from build123d import *

# Parameters (mm, degrees)
F0_W         = 150
F0_H         = 150
F1_DEPTH     = 50
F2_W         = 130.2189305425
F2_H         = 127.2944062948
F3_DEPTH     = 45
F4_T1_DEPTH  = 175.4
F4_T3_DEPTH  = 175.4
F4_T5_DEPTH  = 127.2944062948
F4_T7_DEPTH  = 130.2189305425
F4_T13_DEPTH = 142.9189305425
F4_T17_DEPTH = 139.9944062948
F4_T24_DEPTH = 139.9944062948
F4_T28_DEPTH = 142.9189305425
F4_T35_DEPTH = 139.9944062948
F4_T39_DEPTH = 142.9189305425
F4_T46_DEPTH = 139.9944062948
F4_T50_DEPTH = 142.9189305425


# Not quite as in the source:
# - a fillet or chamfer that OpenCascade refuses, or shapes differently, is made with other operations: its cross-section is extruded or revolved along the edge and cut away or added


with BuildPart() as f1:
    # F0 (on Top) → F1 (new body)
    with BuildSketch(Plane.XY):
        Rectangle(F0_W, F0_H)
    extrude(amount=F1_DEPTH)

    # F2 (on face) → F3 (cut)
    with BuildSketch(Plane.XY.offset(50)):
        with Locations((0.9621791542, 0.0429600477)):
            Rectangle(F2_W, F2_H)
    extrude(amount=-F3_DEPTH, mode=Mode.SUBTRACT)

    # F4: fillet of radius 5.08 on 8 edges, made by hand

    # F4_s2 → F4_t1 (cut)
    with BuildSketch(Plane.YZ.offset(-87.7)):
        with BuildLine():
            ThreePointArc((69.92, 50), (73.5121024484, 48.5121024484), (75, 44.92))
            Line((75, 44.92), (75, 50))
            Line((75, 50), (69.92, 50))
        make_face()
        with BuildLine():
            ThreePointArc((-75, 44.92), (-73.5121024484, 48.5121024484), (-69.92, 50))
            Line((-69.92, 50), (-75, 50))
            Line((-75, 50), (-75, 44.92))
        make_face()
    extrude(amount=F4_T1_DEPTH, mode=Mode.SUBTRACT)

    # F4_s4 → F4_t3 (cut)
    with BuildSketch(Plane.XZ.offset(-87.7)):
        with BuildLine():
            ThreePointArc((-75, 44.92), (-73.5121024484, 48.5121024484), (-69.92, 50))
            Line((-69.92, 50), (-75, 50))
            Line((-75, 50), (-75, 44.92))
        make_face()
        with BuildLine():
            ThreePointArc((75, 44.92), (73.5121024484, 48.5121024484), (69.92, 50))
            Line((69.92, 50), (75, 50))
            Line((75, 50), (75, 44.92))
        make_face()
    extrude(amount=F4_T3_DEPTH, mode=Mode.SUBTRACT)

    # F4_s6 → F4_t5 (cut)
    with BuildSketch(Plane.XZ.offset(-63.6901631951)):
        with BuildLine():
            ThreePointArc((71.1516444254, 50), (67.559541977, 48.5121024484), (66.0716444254, 44.92))
            Line((66.0716444254, 44.92), (66.0716444254, 50))
            Line((66.0716444254, 50), (71.1516444254, 50))
        make_face()
        with BuildLine():
            ThreePointArc((-69.2272861171, 50), (-65.6351836686, 48.5121024484), (-64.1472861171, 44.92))
            Line((-64.1472861171, 44.92), (-64.1472861171, 50))
            Line((-64.1472861171, 50), (-69.2272861171, 50))
        make_face()
    extrude(amount=F4_T5_DEPTH, mode=Mode.SUBTRACT)

    # F4_s8 → F4_t7 (cut)
    with BuildSketch(Plane.YZ.offset(-64.1472861171)):
        with BuildLine():
            ThreePointArc((-68.6842430997, 50), (-65.0921406513, 48.5121024484), (-63.6042430997, 44.92))
            Line((-63.6042430997, 44.92), (-63.6042430997, 50))
            Line((-63.6042430997, 50), (-68.6842430997, 50))
        make_face()
        with BuildLine():
            ThreePointArc((68.7701631951, 50), (65.1780607467, 48.5121024484), (63.6901631951, 44.92))
            Line((63.6901631951, 44.92), (63.6901631951, 50))
            Line((63.6901631951, 50), (68.7701631951, 50))
        make_face()
    extrude(amount=F4_T7_DEPTH, mode=Mode.SUBTRACT)


with BuildPart() as f4_tool11:
    # F4_s12 → F4_t13 (new body)
    with BuildSketch(Plane.YZ.offset(-64.1472861171)):
        with BuildLine():
            ThreePointArc((-68.6842430997, 50), (-65.0921406513, 48.5121024484), (-63.6042430997, 44.92))
            Line((-63.6042430997, 44.92), (-63.6042430997, 50))
            Line((-63.6042430997, 50), (-68.6842430997, 50))
        make_face()
    extrude(amount=F4_T13_DEPTH)

    split(bisect_by=Plane.YZ.offset(66.0716444254), keep=Keep.TOP)


with BuildPart() as f4_tool15:
    # F4_s16 → F4_t17 (new body)
    with BuildSketch(Plane.XZ.offset(76.3042430997)):
        with BuildLine():
            ThreePointArc((71.1516444254, 50), (67.559541977, 48.5121024484), (66.0716444254, 44.92))
            Line((66.0716444254, 44.92), (66.0716444254, 50))
            Line((66.0716444254, 50), (71.1516444254, 50))
        make_face()
    extrude(amount=-F4_T17_DEPTH)

    split(bisect_by=Plane.XZ.offset(63.6042430997), keep=Keep.TOP)


with BuildPart() as f4_tool11_1:
    add(f4_tool11.part)

    # F4_t19: intersect F4_tool15
    add(f4_tool15.part, mode=Mode.INTERSECT)


with BuildPart() as f1_1:
    add(f1.part)

    # F4_t9: cut F4_tool11
    add(f4_tool11_1.part, mode=Mode.SUBTRACT)


with BuildPart() as f4_tool22:
    # F4_s23 → F4_t24 (new body)
    with BuildSketch(Plane.XZ.offset(63.6042430997)):
        with BuildLine():
            ThreePointArc((71.1516444254, 50), (67.559541977, 48.5121024484), (66.0716444254, 44.92))
            Line((66.0716444254, 44.92), (66.0716444254, 50))
            Line((66.0716444254, 50), (71.1516444254, 50))
        make_face()
    extrude(amount=-F4_T24_DEPTH)

    split(bisect_by=Plane.XZ.offset(-63.6901631951), keep=Keep.BOTTOM)


with BuildPart() as f4_tool26:
    # F4_s27 → F4_t28 (new body)
    with BuildSketch(Plane.YZ.offset(78.7716444254)):
        with BuildLine():
            ThreePointArc((68.7701631951, 50), (65.1780607467, 48.5121024484), (63.6901631951, 44.92))
            Line((63.6901631951, 44.92), (63.6901631951, 50))
            Line((63.6901631951, 50), (68.7701631951, 50))
        make_face()
    extrude(amount=-F4_T28_DEPTH)

    split(bisect_by=Plane.YZ.offset(66.0716444254), keep=Keep.TOP)


with BuildPart() as f4_tool22_1:
    add(f4_tool22.part)

    # F4_t30: intersect F4_tool26
    add(f4_tool26.part, mode=Mode.INTERSECT)


with BuildPart() as f1_2:
    add(f1_1.part)

    # F4_t20: cut F4_tool22
    add(f4_tool22_1.part, mode=Mode.SUBTRACT)


with BuildPart() as f4_tool33:
    # F4_s34 → F4_t35 (new body)
    with BuildSketch(Plane.XZ.offset(-63.6901631951)):
        with BuildLine():
            ThreePointArc((-69.2272861171, 50), (-65.6351836686, 48.5121024484), (-64.1472861171, 44.92))
            Line((-64.1472861171, 44.92), (-64.1472861171, 50))
            Line((-64.1472861171, 50), (-69.2272861171, 50))
        make_face()
    extrude(amount=F4_T35_DEPTH)

    split(bisect_by=Plane.XZ.offset(63.6042430997), keep=Keep.TOP)


with BuildPart() as f4_tool37:
    # F4_s38 → F4_t39 (new body)
    with BuildSketch(Plane.YZ.offset(-76.8472861171)):
        with BuildLine():
            ThreePointArc((-68.6842430997, 50), (-65.0921406513, 48.5121024484), (-63.6042430997, 44.92))
            Line((-63.6042430997, 44.92), (-63.6042430997, 50))
            Line((-63.6042430997, 50), (-68.6842430997, 50))
        make_face()
    extrude(amount=F4_T39_DEPTH)

    split(bisect_by=Plane.YZ.offset(-64.1472861171), keep=Keep.BOTTOM)


with BuildPart() as f4_tool33_1:
    add(f4_tool33.part)

    # F4_t41: intersect F4_tool37
    add(f4_tool37.part, mode=Mode.INTERSECT)


with BuildPart() as f1_3:
    add(f1_2.part)

    # F4_t31: cut F4_tool33
    add(f4_tool33_1.part, mode=Mode.SUBTRACT)


with BuildPart() as f4_tool44:
    # F4_s45 → F4_t46 (new body)
    with BuildSketch(Plane.XZ.offset(-76.3901631951)):
        with BuildLine():
            ThreePointArc((-69.2272861171, 50), (-65.6351836686, 48.5121024484), (-64.1472861171, 44.92))
            Line((-64.1472861171, 44.92), (-64.1472861171, 50))
            Line((-64.1472861171, 50), (-69.2272861171, 50))
        make_face()
    extrude(amount=F4_T46_DEPTH)

    split(bisect_by=Plane.XZ.offset(-63.6901631951), keep=Keep.BOTTOM)


with BuildPart() as f4_tool48:
    # F4_s49 → F4_t50 (new body)
    with BuildSketch(Plane.YZ.offset(66.0716444254)):
        with BuildLine():
            ThreePointArc((68.7701631951, 50), (65.1780607467, 48.5121024484), (63.6901631951, 44.92))
            Line((63.6901631951, 44.92), (63.6901631951, 50))
            Line((63.6901631951, 50), (68.7701631951, 50))
        make_face()
    extrude(amount=-F4_T50_DEPTH)

    split(bisect_by=Plane.YZ.offset(-64.1472861171), keep=Keep.BOTTOM)


with BuildPart() as f4_tool44_1:
    add(f4_tool44.part)

    # F4_t52: intersect F4_tool48
    add(f4_tool48.part, mode=Mode.INTERSECT)


with BuildPart() as f1_4:
    add(f1_3.part)

    # F4_t42: cut F4_tool44
    add(f4_tool44_1.part, mode=Mode.SUBTRACT)


solid = f1_4.part
Model file for the job. Use its own axes, mm. A direction names the side the tool comes from. Give positions to 0.01 mm unless a question says otherwise; leave off trailing zeros. Loops run counter-clockwise (first coordinate to the right, second up) from the corner with the lowest first, then second, coordinate; pieces in that order, holes last. Notation, with made-up numbers: (1.5, 7.25) - (24.5, 7.25) arc R16 ccw to (24.5, 14.25) - close; hole circle Ø3 at (12.25, 57.25). An arc over 180 degrees is marked (long way). Use one line per item in the form item = value.
(1) Pull direction X, two halves, no side cores. Call faces 1 (the face through (74.11, 1.05, 47.79)), 2 (the face through (2, 63.69, 25)), 3 (the face through (67.382, -0.911, 48.326)), 4 (the face through (-1, 75, 22)): pulls with the +X half, pulls with the -X half, needs draft (parallel to the pull), parting line crosses it, or undercut.
Determined:
face_1 = pulls with the +X half
face_2 = undercut
face_3 = undercut
face_4 = needs draft
(2) Cut at B-B (y = -41.5). Give the cut face in (x, z), then the cut area to 3 significant figures.
Determined:
outline = (-75, 0) - (75, 0) - (75, 44.92) arc R5.08 ccw to (70.54, 49.96) arc R5.08 ccw to (66.07, 44.92) - (66.07, 5) - (-64.15, 5) - (-64.15, 44.92) arc R5.08 ccw to (-69.23, 50) - (-69.92, 50) arc R5.08 ccw to (-75, 44.92) - close
area = 1,620 mm^2
(3) Cut at A-A (z = 41.5). Give the cut face in (x, y), then the cut area to 3 significant figures.
Determined:
outline = (-75, -75) - (75, -75) - (75, 75) - (-75, 75) - close; hole (-64.15, -63.6) - (66.07, -63.6) - (66.07, 63.69) - (-64.15, 63.69) - close
area = 5,920 mm^2
(4) Cut at C-C (x = 39). Give the cut face in (y, z).
Determined:
outline = (-75, 0) - (75, 0) - (75, 44.92) arc R5.08 ccw to (69.92, 50) - (68.77, 50) arc R5.08 ccw to (63.69, 44.92) - (63.69, 5) - (-63.6, 5) - (-63.6, 44.92) arc R5.08 ccw to (-68.68, 50) - (-69.92, 50) arc R5.08 ccw to (-75, 44.92) - close
(5) Drill centre lines: L1, parallel to X at y = 10, z = 17.5; L2, parallel to Y at x = -18, z = 20; L3, parallel to Z at x = -18.5, y = -35.5. Where is each one in solid material? Low to high.
Determined:
L1 = -75 to -64.15, 66.07 to 75
L2 = -75 to -63.6, 63.69 to 75
L3 = 0 to 5
(6) 3-axis set-ups, long thin cutter, end or side, ignore diameter. For faces 5 (the face through (0, 1, 5)), 6 (the face through (75, -1, 22)): which of +Z, -Z, +X, -X, +Y, -Y reach the whole face in a straight line?
Determined:
face_5 = +Z
face_6 = +Z, -Z, +X, +Y, -Y
(7) Drop flat-ended pins along their axis: P1, Ø4, axis at x = -43.5, y = -57, coming from the -Z side; P2, Ø3, axis at x = -59, y = 41.5, coming from the +Z side. Give the stop position or say it passes through.
Determined:
P1 = 0
P2 = 5
